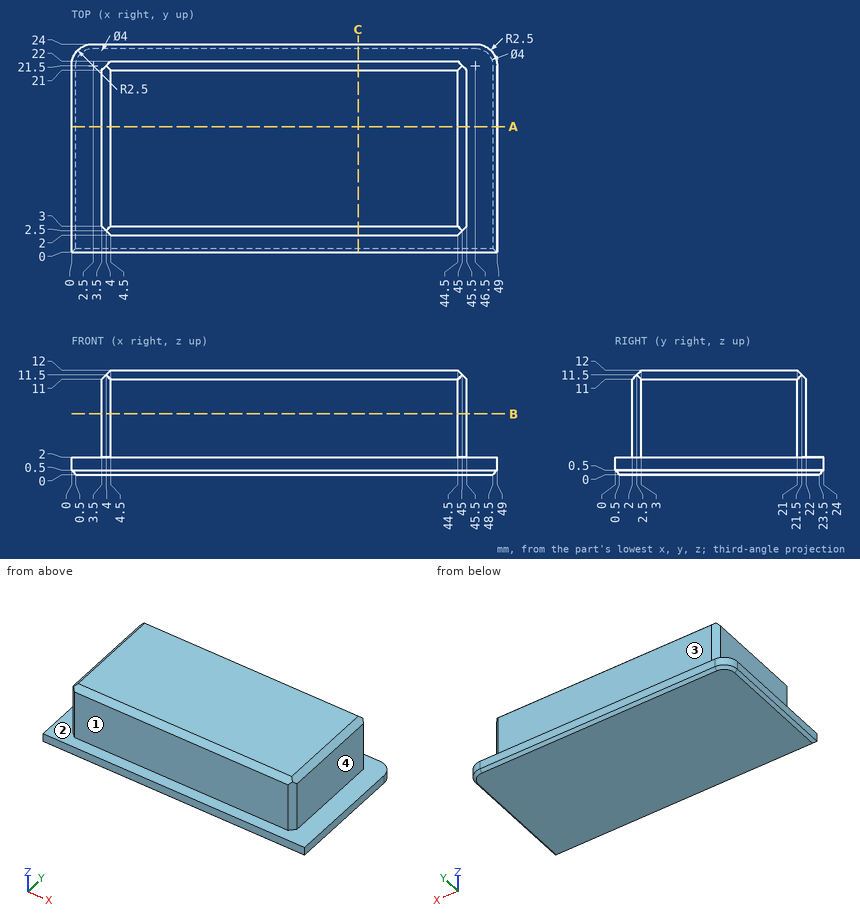
For this review, use the dimensioned drawing (mm, ordinates from the lowest corner) and the shaded views. A direction names the side the tool comes from. Give positions to 0.01 mm unless a question says otherwise; leave off trailing zeros. Write each loop counter-clockwise with the first axis right and the second up, starting at its lowest first coordinate (ties: lowest second). Pieces come first, ordered by that corner, then holes.
(1) Consider section B-B, the plane z = 7. Give the boundary of the cut face in (x, y), and give its area (3 significant figures).
(2) Consider section C-C, the plane x = 33. Give the boundary of the cut face in (y, z).
(3) Tool access review of the marked faces 1, 2, 3 and 4: name each direction out of +Z, -Z, +X, -X, +Y, -Y from which nothing blocks a thin tool from reaching the whole face with its end or side.
(4) Consider section A-A, the plane y = 14.5. Give the boundary of the cut face in (x, z).
(5) To check wall thickness, follow L1, parallel to Y at x = 29.5, z = 11.5; L2, parallel to X at y = 9.25, z = 8.25; L3, parallel to Y at x = 40, z = 8.5. State the ranges of each line that lie inside material, in increasing order.
(6) For P1, Ø7, axis at y = 16, z = 6, coming from the -X side; P2, Ø2.5, axis at x = 20.5, z = 4.5, coming from the +Y side; P3, Ø4.5, axis at x = 18.5, z = 5.5, coming from the -Y side, all flat-tipped, find the tip position at first contact; note any pin that passes through.
Returned:
1. outline: (3.5, 3) - (4.5, 2) - (44.5, 2) - (45.5, 3) - (45.5, 21) - (44.5, 22) - (4.5, 22) - (3.5, 21) - close
1. area: 838 mm2
2. outline: (0, 0.5) - (0.5, 0) - (23.5, 0) - (24, 0.5) - (24, 2) - (22, 2) - (22, 11) - (21, 12) - (3, 12) - (2, 11) - (2, 2) - (0, 2) - close
3. face 1: +Z, +X, -X, -Y
3. face 2: +Z
3. face 3: +Z, +X, -X, +Y
3. face 4: +Z, +X, +Y, -Y
4. outline: (0, 0.5) - (0.5, 0) - (48.5, 0) - (49, 0.5) - (49, 2) - (45.5, 2) - (45.5, 11) - (44.5, 12) - (4.5, 12) - (3.5, 11) - (3.5, 2) - (0, 2) - close
5. L1: y = 2.5 to 21.5
5. L2: x = 3.5 to 45.5
5. L3: y = 2 to 22
6. P1: stops at x = 3.5
6. P2: stops at y = 22
6. P3: stops at y = 2
